Autodesk Inventor part; units mm, degrees
ref_plane "YZ Plane" through (0, 0, 0) normal (1, 0, 0) x (0, 1, 0)
ref_plane "XZ Plane" through (0, 0, 0) normal (0, 1, 0) x (-1, 0, 0)
ref_plane "XY Plane" through (0, 0, 0) normal (0, 0, 1) x (1, 0, 0)
sketch "Sketch1" plane through (0, 0, 0) normal (0, 1, 0) x (-1, 0, 0)
  line L0 (0, 0) -> (18.5658, -69.2885)
  circle A0 centre (25.8819, -96.5926) radius 5
  arc A1 (24.729, -72.9816) -> (15.0747, -75.5678) centre (19.8599, -74.1181) ccw
  line L1 (30.6777, -95.1782) -> (24.6448, -72.6673)
  line L2 (21.0523, -97.8867) -> (14.9907, -75.2542)
  circle A2 centre (0, -103.5276) radius 11.6229
  line L3 (21.0523, -97.8867) -> (25.8819, -96.5926)
  arc A3 (-25.8819, -96.5926) -> (26.7197, -101.5219) centre (0, -103.5276) ccw
  circle A4 centre (0, -103.5276) radius 39.9
  arc A5 (57.9067, -50.8394) -> (50.8389, -57.9063) centre (54.2582, -54.2582) ccw
  line L4 (67.1751, -74.2462) -> (50.6094, -57.6767)
  line L5 (74.1567, -67.0879) -> (57.6767, -50.6094)
  circle A6 centre (70.7107, -70.7107) radius 5
  circle A7 centre (51.7638, -89.6575) radius 11.6229
  arc A8 (75.5684, -15.0748) -> (72.9809, -24.7289) centre (74.1181, -19.8599) ccw
  line L6 (95.2985, -30.7115) -> (72.6673, -24.6448)
  line L7 (97.7655, -21.0214) -> (75.2542, -14.9907)
  circle A9 centre (96.5926, -25.8819) radius 5
  circle A10 centre (89.6575, -51.7638) radius 11.6229
  arc A11 (72.9816, 24.729) -> (75.5678, 15.0747) centre (74.1181, 19.8599) ccw
  line L8 (97.8867, 21.0523) -> (75.2542, 14.9907)
  line L9 (95.1782, 30.6777) -> (72.6673, 24.6448)
  circle A12 centre (96.5926, 25.8819) radius 5
  circle A13 centre (103.5276, 0) radius 11.6229
  arc A14 (50.8394, 57.9067) -> (57.9063, 50.8389) centre (54.2582, 54.2582) ccw
  line L10 (74.2462, 67.1751) -> (57.6767, 50.6094)
  line L11 (67.0879, 74.1567) -> (50.6094, 57.6767)
  circle A15 centre (70.7107, 70.7107) radius 5
  circle A16 centre (89.6575, 51.7638) radius 11.6229
  arc A17 (15.0748, 75.5684) -> (24.7289, 72.9809) centre (19.8599, 74.1181) ccw
  line L12 (30.7115, 95.2985) -> (24.6448, 72.6673)
  line L13 (21.0214, 97.7655) -> (14.9907, 75.2542)
  circle A18 centre (25.8819, 96.5926) radius 5
  circle A19 centre (51.7638, 89.6575) radius 11.6229
  arc A20 (-24.729, 72.9816) -> (-15.0747, 75.5678) centre (-19.8599, 74.1181) ccw
  line L14 (-21.0523, 97.8867) -> (-14.9907, 75.2542)
  line L15 (-30.6777, 95.1782) -> (-24.6448, 72.6673)
  circle A21 centre (-25.8819, 96.5926) radius 5
  circle A22 centre (0, 103.5276) radius 11.6229
  arc A23 (-57.9067, 50.8394) -> (-50.8389, 57.9063) centre (-54.2582, 54.2582) ccw
  line L16 (-67.1751, 74.2462) -> (-50.6094, 57.6767)
  line L17 (-74.1567, 67.0879) -> (-57.6767, 50.6094)
  circle A24 centre (-70.7107, 70.7107) radius 5
  circle A25 centre (-51.7638, 89.6575) radius 11.6229
  arc A26 (-75.5684, 15.0748) -> (-72.9809, 24.7289) centre (-74.1181, 19.8599) ccw
  line L18 (-95.2985, 30.7115) -> (-72.6673, 24.6448)
  line L19 (-97.7655, 21.0214) -> (-75.2542, 14.9907)
  circle A27 centre (-96.5926, 25.8819) radius 5
  circle A28 centre (-89.6575, 51.7638) radius 11.6229
  arc A29 (-72.9816, -24.729) -> (-75.5678, -15.0747) centre (-74.1181, -19.8599) ccw
  line L20 (-97.8867, -21.0523) -> (-75.2542, -14.9907)
  line L21 (-95.1782, -30.6777) -> (-72.6673, -24.6448)
  circle A30 centre (-96.5926, -25.8819) radius 5
  circle A31 centre (-103.5276, 0) radius 11.6229
  arc A32 (-50.8394, -57.9067) -> (-57.9063, -50.8389) centre (-54.2582, -54.2582) ccw
  line L22 (-74.2462, -67.1751) -> (-57.6767, -50.6094)
  line L23 (-67.0879, -74.1567) -> (-50.6094, -57.6767)
  circle A33 centre (-70.7107, -70.7107) radius 5
  circle A34 centre (-89.6575, -51.7638) radius 11.6229
  arc A35 (-15.0748, -75.5684) -> (-24.7289, -72.9809) centre (-19.8599, -74.1181) ccw
  line L24 (-30.7115, -95.2985) -> (-24.6448, -72.6673)
  line L25 (-21.0214, -97.7655) -> (-14.9907, -75.2542)
  circle A36 centre (-25.8819, -96.5926) radius 5
  circle A37 centre (-51.7638, -89.6575) radius 11.6229
  circle A38 centre (0, 0) radius 5
  circle A39 centre (0, -103.5276) radius 2
  circle A40 centre (0, -76.7327) radius 5
  circle A41 centre (0, -103.5276) radius 32.5
  circle A42 centre (0, -76.7327) radius 3
  circle A43 centre (0, -103.5276) radius 2
  arc A44 (24.6448, -72.6673) -> (-14.9907, -75.2542) centre (0, 0) ccw
  arc A45 (-4.9973, -76.5698) -> (4.9973, -76.5698) centre (0, 0) ccw
  line L26 (0, 0) -> (0, -63.6276)
  line L27 (0, -71.0276) -> (0, -103.5276)
  arc A46 (21.0199, -97.7659) -> (21.0214, -97.7655) centre (0, 0) ccw
  arc A47 (30.6777, -95.1782) -> (-21.0214, -97.7655) centre (0, 0) ccw
  point P0 (0, 0)
  point P1 (0, 0)
  point P2 (50.7227, -50.7227)
  point P3 (73.9009, -74.5607)
  point P4 (69.2885, -18.5658)
  point P5 (101.2804, -27.621)
  point P6 (69.2885, 18.5658)
  point P7 (101.5219, 26.7197)
  point P8 (50.7227, 50.7227)
  point P9 (74.5607, 73.9009)
  point P10 (18.5658, 69.2885)
  point P11 (27.621, 101.2804)
  point P12 (-18.5658, 69.2885)
  point P13 (-26.7197, 101.5219)
  point P14 (-50.7227, 50.7227)
  point P15 (-73.9009, 74.5607)
  point P16 (-69.2885, 18.5658)
  point P17 (-101.2804, 27.621)
  point P18 (-69.2885, -18.5658)
  point P19 (-101.5219, -26.7197)
  point P20 (-50.7227, -50.7227)
  point P21 (-74.5607, -73.9009)
  point P22 (-18.5658, -69.2885)
  point P23 (-27.621, -101.2804)
  point P24 (40.2917, -91.5236)
  point P25 (59.1159, -80.6555)
  point P26 (67.0867, -74.1578)
  point P27 (74.1567, -67.0879)
  point P28 (80.6555, -59.1159)
  point P29 (91.5236, -40.2917)
  point P30 (95.1777, -30.6791)
  point P31 (97.7655, -21.0214)
  point P32 (99.4077, -10.8682)
  point P33 (99.4077, 10.8682)
  point P34 (97.7659, 21.0199)
  point P35 (95.1782, 30.6777)
  point P36 (91.5236, 40.2917)
  point P37 (80.6555, 59.1159)
  point P38 (74.1578, 67.0867)
  point P39 (67.0879, 74.1567)
  point P40 (59.1159, 80.6555)
  point P41 (40.2917, 91.5236)
  point P42 (30.6791, 95.1777)
  point P43 (21.0214, 97.7655)
  point P44 (10.8682, 99.4077)
  point P45 (-10.8682, 99.4077)
  point P46 (-21.0199, 97.7659)
  point P47 (-30.6777, 95.1782)
  point P48 (-40.2917, 91.5236)
  point P49 (-59.1159, 80.6555)
  point P50 (-67.0867, 74.1578)
  point P51 (-74.1567, 67.0879)
  point P52 (-80.6555, 59.1159)
  point P53 (-91.5236, 40.2917)
  point P54 (-95.1777, 30.6791)
  point P55 (-97.7655, 21.0214)
  point P56 (-99.4077, 10.8682)
  point P57 (-99.4077, -10.8682)
  point P58 (-97.7659, -21.0199)
  point P59 (-95.1782, -30.6777)
  point P60 (-91.5236, -40.2917)
  point P61 (-80.6555, -59.1159)
  point P62 (-74.1578, -67.0867)
  point P63 (-67.0879, -74.1567)
  point P64 (-59.1159, -80.6555)
  point P65 (-40.2917, -91.5236)
  point P66 (-30.6791, -95.1777)
  point P67 (-21.0214, -97.7655)
  point P68 (-10.8682, -99.4077)
  point P69 (10.8682, -99.4077)
  point P70 (-10.8682, -99.4077)
  point P71 (10.8682, -99.4077)
  dimension "d6" = 79.8
  dimension "d11" = 65
  dimension "d4" = 10
  dimension "d5" = 10
  dimension "d7" = 360
  dimension "d8" = 10
  dimension "d9" = 4
  dimension "d10" = 10
  dimension "d12" = 6
extrude "Extrusion1" add sketch "Sketch1" along normal blind 10 contours A41 L1 A0 L2 A1 | A1 L2 A46 A2 L27 A40 A41 | A41 L27 A40 A2 A46 L25 A35 | A35 A44 A41 | L2 A1 | A41 A46 L1 | A35 L25 A36 L24 A41 A44 | A46 A41 L24 A36 A3 A0 | A46 A0 | A0 L3 A46 | L27 A42 A45 A40 | A40 A45 A42 L27 | L24 A46 A41 | A46 L3 A0 | A0 A3 A36 A46 A2 | A40 L27 A42 A45 | A45 A42 L27 A40 | A46 A36 | A36 A3 A46 | A46 A3 A36 L24 | A46 L27 A2 | A2 A46 | A2 L27 A46
properties part number "SC-1-02-Circle Arc Cover"
Could you check a few things on this model? Use its own coordinates, in mm. Coordinates: 2 decimals unless noted, no trailing zeros. Write each loop counter-clockwise with the first axis right and the second up, starting at its lowest first coordinate (ties: lowest second). Pieces come first, ordered by that corner, then holes. Notation, with made-up numbers: (-8, 29) -> (40, 29) arc R10 ccw to (40, 33) -> close; hole circle Ø4 at (50.25, -6.5). An arc over 180 degrees is marked (long way). One line per question, with ' | ' between items. Start each with the question number.
1. If we section it at A-A (y = 7.75): Please give me the cut outline in (x, z).
2. If we section it at B-B (x = 8.5): Please give me the cut outline in (y, z), and give its area (3 significant figures).
3. If we section it at C-C (z = -90): Please give me the cut outline in (x, y).
4. Will these pins go through, and if not, where does the flat tip stop? P1, Ø3, axis at x = -10.5, y = 3.5, coming from the -Z side; P2, Ø1, axis at x = 18.5, y = 4.5, coming from the -Z side; P3, Ø3, axis at y = 6, z = -81, coming from the -X side.
5. Please list where these lines run through material, in increasing order: line 1 along Z through (x, y) = (0, 7.75); line 2 along X through (y, z) = (8, -104); line 3 along X through (y, z) = (7, -77.5).
Return value:
1) outline: circle Ø65 at (0, -103.53); hole circle Ø6 at (0, -76.73); hole circle Ø4 at (0, -103.53)
2) outline: (0, -134.9) -> (10, -134.9) -> (10, -72.16) -> (0, -72.16) -> close | area: 627 mm²
3) outline: (-29.55, 0) -> (29.55, 0) -> (29.55, 10) -> (-29.55, 10) -> close
4) P1: stops at z = -134.76 | P2: stops at z = -130.59 | P3: stops at x = -24.78
5) line 1: z = -136.03 to -105.53, -101.53 to -79.73, -73.73 to -71.03 | line 2: x = -32.5 to -1.94, 1.94 to 32.5 | line 3: x = -19.46 to -2.9, 2.9 to 19.46
